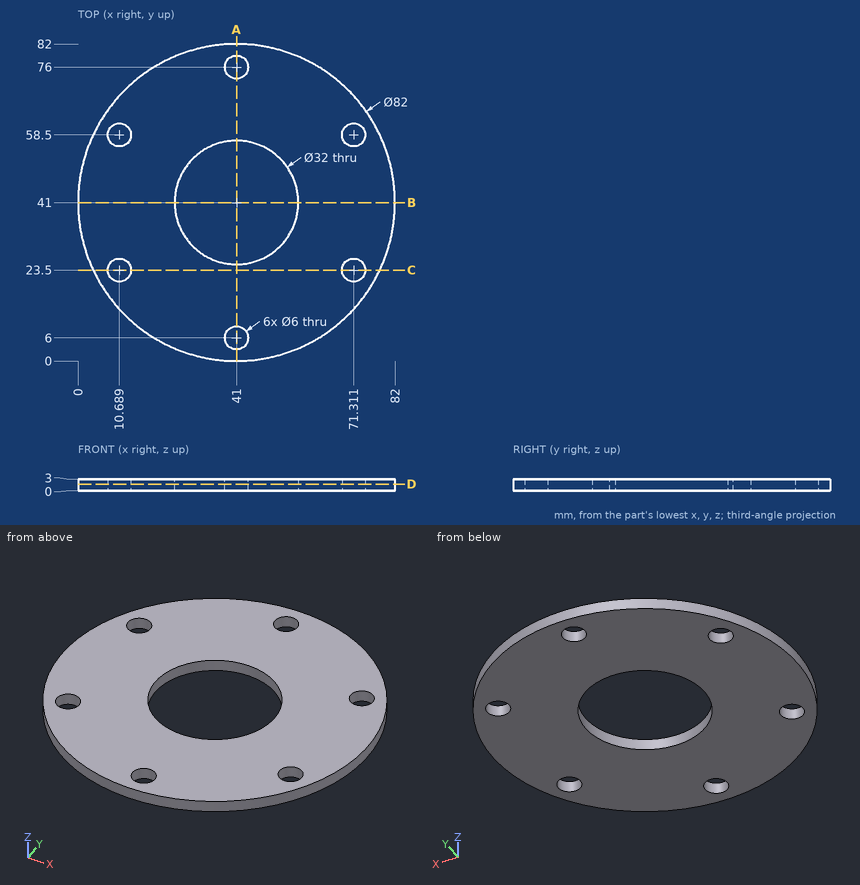
Verification items for this drawing (mm, ordinates from the low corner). Coordinates: 2 decimals unless noted, no trailing zeros. Order: outer loops, then holes, each group sorted by start corner. A loop starts at its lowest first (then second) coordinate and runs counter-clockwise, first axis right, second up. Notation, with made-up numbers: (72, -4.5) - (129, -4.5) arc R28 ccw to (129, 24.5) - close; hole circle Ø9 at (11.25, -9.75). An arc over 180 degrees is marked (long way). Answer as a JSON object with one key per item and string values. Group by question number.
Item 1: Sectioned sample at C-C, the plane y = 23.5. Record the cut outline in (x, z), and give its area (3 significant figures).
Item 2: Sectioned sample at D-D, the plane z = 1.7. Record the cut outline in (x, y).
Item 3: Scan lines: probe 1 along Y at (x, z) = (41, 2.05); probe 2 along X at (y, z) = (58, 2.5); probe 3 along Y at (x, z) = (11, 2.65). Record each from-to range of solid material in increasing order.
Item 4: Sectioned sample at B-B, the plane y = 41. Record the cut outline in (x, z), and give its area (3 significant figures).
Item 5: Sectioned sample at A-A, the plane x = 41. Record the cut outline in (y, z), and give its area (3 significant figures).
Item 6: Depth check by flat-ended pin: pin 1 Ø1 at (x, z) = (47.5, 1.5) entering from -Y; pin 2 Ø1.5 at (x, z) = (35.5, 1) entering from +Y. Enter the tip coordinate at first touch or a pass-through.
Resolved:
{
 "1": {"outline": "(3.92, 0) - (7.69, 0) - (7.69, 3) - (3.92, 3) - close; (13.69, 0) - (68.31, 0) - (68.31, 3) - (13.69, 3) - close; (74.31, 0) - (78.08, 0) - (78.08, 3) - (74.31, 3) - close", "area": "186 mm^2"},
 "2": {"outline": "circle Ø82 at (41, 41); hole circle Ø6 at (10.69, 23.5); hole circle Ø6 at (10.69, 58.5); hole circle Ø32 at (41, 41); hole circle Ø6 at (41, 6); hole circle Ø6 at (41, 76); hole circle Ø6 at (71.31, 23.5); hole circle Ø6 at (71.31, 58.5)"},
 "3": {"probe 1": "0 to 3, 9 to 25, 57 to 73, 79 to 82", "probe 2": "3.69 to 7.73, 13.65 to 68.35, 74.27 to 78.31", "probe 3": "13.05 to 20.52, 26.48 to 55.52, 61.48 to 68.95"},
 "4": {"outline": "(0, 0) - (25, 0) - (25, 3) - (0, 3) - close; (57, 0) - (82, 0) - (82, 3) - (57, 3) - close", "area": "150 mm^2"},
 "5": {"outline": "(0, 0) - (3, 0) - (3, 3) - (0, 3) - close; (9, 0) - (25, 0) - (25, 3) - (9, 3) - close; (57, 0) - (73, 0) - (73, 3) - (57, 3) - close; (79, 0) - (82, 0) - (82, 3) - (79, 3) - close", "area": "114 mm^2"},
 "6": {"pin 1": "y = 0.44", "pin 2": "y = 81.72"}
}
